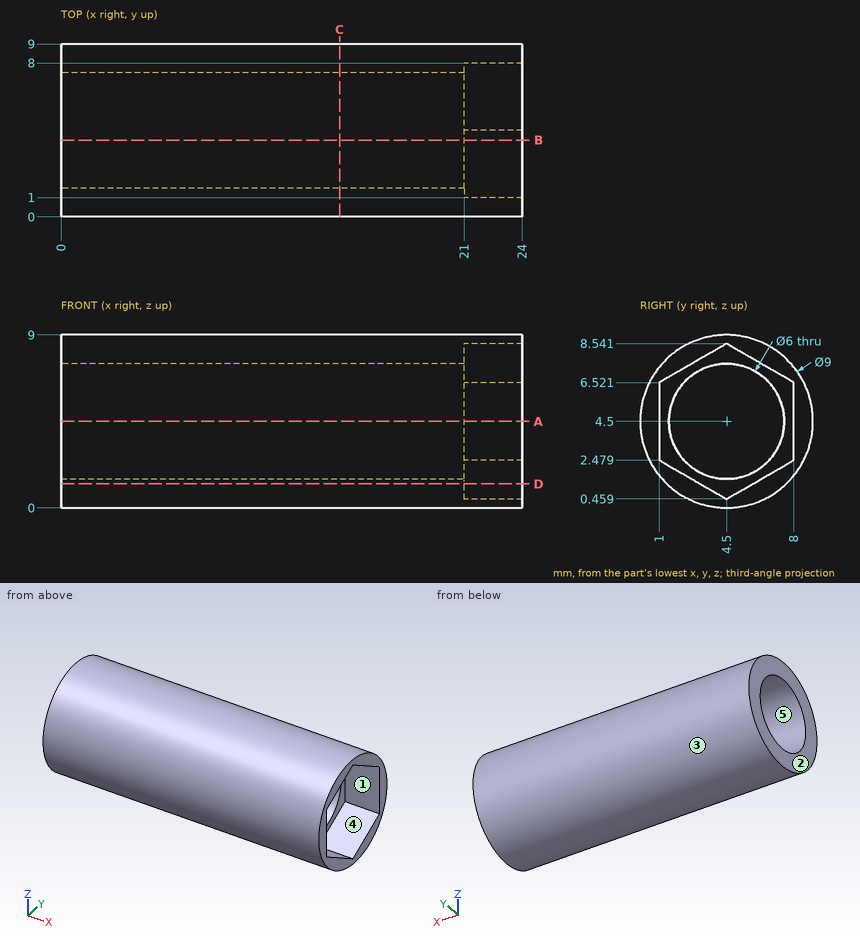
Design review of the part shown in the three views and the two pictorial views. Dimensions are in mm from the part's minimum x, y and z. A direction names the side the tool comes from. Round coordinates to 2 decimals unless told otherwise and drop trailing zeros. Write each loop counter-clockwise with the first axis right and the second up, starting at its lowest first coordinate (ties: lowest second). Pieces come first, ordered by that corner, then holes.
Item 1: We need section C-C on x = 14.5. Write out the cut boundary in (y, z).
Item 2: We need section B-B on y = 4. Write out the cut boundary in (x, z).
Item 3: For the marked faces 4 and 5, list the 3-axis set-ups (+Z, -Z, +X, -X, +Y, -Y) from which the entire face can be reached by the end or side of a thin tool; tool diameter is ignored.
Item 4: For probe 1 along Y at (x, z) = (15.75, 4.5); probe 2 along X at (y, z) = (2, 6.25); probe 3 along Z at (x, y) = (19.5, 4.75), list the stretches that pass through material, from the lowest coordinate up.
Item 5: We need section D-D on z = 1.25. Write out the cut boundary in (x, y), and give its area (3 significant figures).
Item 6: The part is to be moulded in two halves that separate along Z. For the marked faces 1, 2 and 3, say which applies: +Z half, -Z half, draft (parallel to the pull), parting line (faces both ways), or undercut.
Item 7: We need section A-A on z = 4.5. Write out the cut boundary in (x, y).
Item 8: Clearance check with flat-ended pins moving along their axes: pin 1 Ø3 at (x, z) = (19, 7) entering from +Y; pin 2 Ø1.5 at (y, z) = (1.5, 4) entering from -X; pin 3 Ø3.5 at (y, z) = (6, 5.5) entering from +X; pin 4 Ø4 at (x, y) = (8.5, 8) entering from +Z. State where each tip first meets the part, or that it passes through.
Returned:
1. outline: circle Ø9 at (4.5, 4.5); hole circle Ø6 at (4.5, 4.5)
2. outline: (0, 0.03) - (24, 0.03) - (24, 0.75) - (21, 0.75) - (21, 1.54) - (0, 1.54) - close; (0, 7.46) - (21, 7.46) - (21, 8.25) - (24, 8.25) - (24, 8.97) - (0, 8.97) - close
3. face 4: +X
3. face 5: +X, -X
4. probe 1: y = 0 to 1.5, 7.5 to 9
4. probe 2: x = 0 to 21
4. probe 3: z = 0.01 to 1.51, 7.49 to 8.99
5. outline: (0, 1.39) - (24, 1.39) - (24, 3.13) - (21, 3.13) - (21, 5.87) - (24, 5.87) - (24, 7.61) - (0, 7.61) - close
5. area: 141 mm2
6. face 1: undercut
6. face 2: draft
6. face 3: parting line
7. outline: (0, 0) - (24, 0) - (24, 1) - (21, 1) - (21, 1.5) - (0, 1.5) - close; (0, 7.5) - (21, 7.5) - (21, 8) - (24, 8) - (24, 9) - (0, 9) - close
8. pin 1: stops at y = 8.89
8. pin 2: stops at x = 0
8. pin 3: stops at x = 21
8. pin 4: stops at z = 8.74
